Input: part model. Units: mm. Frame: model coordinates. A direction names the side the tool comes from. Round coordinates to 2 decimals unless told otherwise and drop trailing zeros. Order: outer loops, then holes, each group sorted by start corner. A loop starts at its lowest first (then second) coordinate and runs counter-clockwise, first axis right, second up. Notation, with made-up numbers: (1.25, 53.5) -> (13.25, 53.5) arc R22 cw to (13.25, 86.5) -> close; hole circle Ø1 at (32, -25). An arc over 180 degrees is marked (long way). Use a Markdown table: item, result.
from build123d import *

# Parameters (mm, degrees)
EXTRUDE_1_DEPTH = 10


with BuildPart() as part:
    # 草图1 → 凸台-拉伸1 (new, symmetric)
    with BuildSketch(Plane(origin=(0, 0, 0), x_dir=(1, 0, 0), z_dir=(0, 1, 0))):
        Polygon((2.684678752, 0), (1.342339376, 2.325), (-1.342339376, 2.325), (-2.684678752, 0), (-1.342339376, -2.325), (1.342339376, -2.325), align=None)
    extrude(amount=EXTRUDE_1_DEPTH, both=True)

    # 草图2 → M3 螺纹孔1 (revolve, cut)
    with BuildSketch(Plane(origin=(0, -10, 0), x_dir=(0, 0, -1), z_dir=(1, 0, 0))):
        Polygon((0, 0), (0, 8.251075774), (1.25, 7.5), (1.25, 0), align=None)
    hole_wizard_m3_1 = revolve(axis=Axis((0, -16.35, 0), (0, 1, 0)), mode=Mode.SUBTRACT)

    # 镜向1: M3 螺纹孔1 across plane
    add(hole_wizard_m3_1.mirror(Plane.ZX), mode=Mode.SUBTRACT)


solid = part.part
1) Set-up query: faces 1 (the cylindrical face through (1.22, 6.3, 0.27)), 2 (the cylindrical face through (1.22, -6.3, 0.27)), 3 (the flat face through (1, -10, -1)). Return all of +Z, -Z, +X, -X, +Y, -Y with unobstructed straight access to the full face (end or side cutting, diameter ignored); none if empty.
Results found:
| item | result |
|---|---|
| face 1 | +Y |
| face 2 | -Y |
| face 3 | +Z, -Z, +X, -X, -Y |
2) Cut plane C-C on z = 1.8. Return loops of the section in (x, y), and give its area (3 significant figures).
Results found:
| item | result |
|---|---|
| outline | (-1.65, -10) -> (1.65, -10) -> (1.65, 10) -> (-1.65, 10) -> close |
| area | 65.8 mm² |
3) Line query: L1, parallel to Z at x = 0, y = 4 (3 decimals); L2, parallel to X at y = 4.25, z = 0.9; L3, parallel to X at y = -4, z = 0.7. Output: solid intervals per line, ascending. Write a range as [from, to].
Results found:
| item | result |
|---|---|
| L1 | z = [-2.325, -1.25], [1.25, 2.325] |
| L2 | x = [-2.17, -0.87], [0.87, 2.17] |
| L3 | x = [-2.28, -1.04], [1.04, 2.28] |
4) Cut plane B-B on x = 1.6. Return loops of the section in (y, z), and give its area (3 significant figures).
Results found:
| item | result |
|---|---|
| outline | (-10, -1.88) -> (10, -1.88) -> (10, 1.88) -> (-10, 1.88) -> close |
| area | 75.1 mm² |
5) Pull-direction query (X, two-part tool) for faces 4 (the conical face through (0.21, -1.88, 0.05)), 5 (the flat face through (1, 10, -1)), 6 (the flat face through (-2.004, 0.14, -1.179)); classes: +X half, -X half, draft (parallel to the pull), parting line (faces both ways), or undercut.
Results found:
| item | result |
|---|---|
| face 4 | undercut |
| face 5 | draft |
| face 6 | -X half |
6) Pin query (flat end, axial travel): pin 1 Ø1.5 at (x, z) = (0, 0) entering from +Y; pin 2 Ø1.5 at (x, y) = (-1.5, 4) entering from +Z (3 decimals). Return the tip coordinate at first contact, or that it passes through.
Results found:
| item | result |
|---|---|
| pin 1 | stops at y = 2.2 |
| pin 2 | stops at z = 2.325 |
7) Cut plane A-A on y = 6.75. Return loops of the section in (x, z) (3 decimals), and give its area (3 significant figures).
Results found:
| item | result |
|---|---|
| outline | (-2.685, 0) -> (-1.342, -2.325) -> (1.342, -2.325) -> (2.685, 0) -> (1.342, 2.325) -> (-1.342, 2.325) -> close; hole circle Ø2.5 at (0, 0) |
| area | 13.8 mm² |
